Here's how the part is built. I have some questions about the finished solid (model axes, mm). Coordinates: 2 decimals unless noted, no trailing zeros. Loops run counter-clockwise (first coordinate to the right, second up) from the corner with the lowest first, then second, coordinate; pieces in that order, holes last. Notation, with made-up numbers: M -14.5,34.5 L 32.5,34.5 A13 cw 32.5,58.5 Z; hole C -26,28.25 d10. An arc over 180 degrees is marked long. Use one line per item in the form item = value. Start each with the question number.
(1) Imagine slicing it at A-A, the plane z = 0.9. State how many separate pieces and enclosed holes the cut face has, and give its area (3 significant figures).
(2) Imagine slicing it at C-C, the plane y = 24.5. Please give me the cut outline in (x, z).
(3) Please list where these lines run through material, in increasing order: L1, parallel to Y at x = 40, z = 0.1; L2, parallel to X at y = 17, z = 0.95; L3, parallel to X at y = 50.8, z = 0.7.
(4) Imagine slicing it at B-B, the plane x = 47.5. Please give me the cut outline in (y, z).
Autodesk Inventor part; units mm, degrees
ref_plane "YZ Plane" through (0, 0, 0) normal (1, 0, 0) x (0, 1, 0)
ref_plane "XZ Plane" through (0, 0, 0) normal (0, 1, 0) x (-1, 0, 0)
ref_plane "XY Plane" through (0, 0, 0) normal (0, 0, 1) x (1, 0, 0)
sketch "Sketch1" plane through (0, 0, 0) normal (0, 0, 1) x (1, 0, 0)
  line L0 (0, 10.0078) -> (0, -10.7712)
  line L1 (-20.5368, 0) -> (25.7294, 0)
  line L2 (0, 0) -> (-9.8402, -9.8402)
  line L3 (0, 0) -> (13.9161, 0) construction
  line L4 (0, 0) -> (-23.2805, 23.2805)
  circle A0 centre (0, 0) radius 66.675
  point P0 (-16.1645, 16.1645)
  point P1 (-41.3092, 41.3092)
  point P2 (-41.3092, -41.3092)
  point P3 (-16.1645, -16.1645)
  point P4 (16.1645, 16.1645)
  point P5 (41.3092, 41.3092)
  point P6 (41.3092, -41.3092)
  point P7 (16.1645, -16.1645)
  point P8 (26.5906, 50.8)
  point P9 (-26.5906, 50.8)
  point P10 (23.2805, 23.2805)
  point P11 (16.1645, 16.1645)
  point P12 (26.5906, -50.8)
  point P13 (-26.5906, -50.8)
  dimension "d1" = 45
  dimension "d56" = 22.86
  dimension "d58" = 35.56
  dimension "d67" = 53.1812
  dimension "d68" = 101.6
  dimension "d85" = 133.35
extrude "Extrusion1" add sketch "Sketch1" along normal blind 1.5875
hole "Hole1" at (-16.1645, 16.1645, 0) at (-41.3092, 41.3092, 0) at (-41.3092, -41.3092, 0) at (-16.1645, -16.1645, 0) at (41.3092, 41.3092, 0) at (16.1645, 16.1645, 0) at (16.1645, -16.1645, 0) at (41.3092, -41.3092, 0) direction (0, 0, 1) diameter 3.302 end through all
sketch "Sketch2" plane through (0, 0, 0) normal (0, 0, -1) x (-1, 0, 0)
  line L0 (0, -11.8713) -> (0, 16.3095)
  line L1 (-16.3095, 0) -> (16.3095, 0)
  point P0 (23.2805, -60.3987)
  point P1 (0, 0)
  point P2 (26.5906, 50.8)
  point P3 (-26.5906, 50.8)
  point P4 (26.5906, -50.8)
  point P5 (-26.5906, -50.8)
  dimension "d69" = 53.1812
  dimension "d70" = 101.6
hole "Hole3" at (-26.5906, -50.8, 0) at (26.5906, -50.8, 0) at (26.5906, 50.8, 0) at (-26.5906, 50.8, 0) direction (0, 0, 1) diameter 2.6416 end through all
properties part number "BaseBottom"
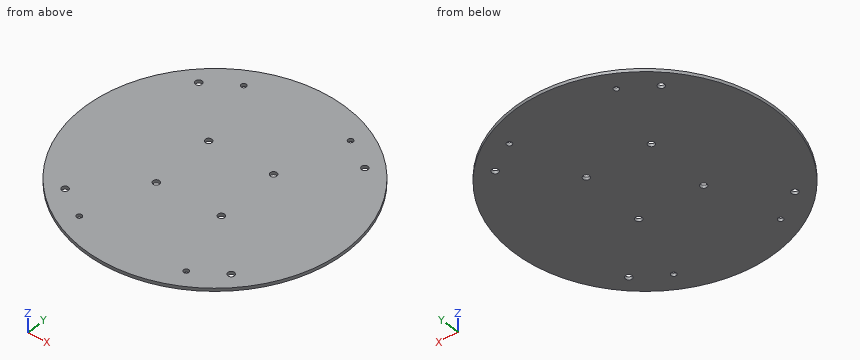
Answer:
q1.separate_pieces = 1
q1.enclosed_holes = 12
q1.area = 13,900 mm²
q2.outline = M -62.01,0 L 62.01,0 L 62.01,1.59 L -62.01,1.59 Z
q3.L1 = -53.34 to -42.32, -40.3 to 40.3, 42.32 to 53.34
q3.L2 = -64.47 to -17.59, -14.74 to 14.74, 17.59 to 64.47
q3.L3 = -43.18 to -27.91, -25.27 to 25.27, 27.91 to 43.18
q4.outline = M -46.79,0 L 46.79,0 L 46.79,1.59 L -46.79,1.59 Z
